Read the model definition and answer for the solid it produces. Units are mm, in the model's axes. Face numbers are marked on the shaded views. A direction names the side the tool comes from. Coordinates: 2 decimals unless noted, no trailing zeros. Write each loop counter-clockwise with the first axis right and the second up, starting at its lowest first coordinate (ties: lowest second). Pieces come first, ordered by that corner, then holes.
(1) The part is cut by section A-A, the plane x = 0. Determine the outline of the cut face in (y, z), and give its area (3 significant figures).
(2) The part is cut by section C-C, the plane z = 20. Determine the outline of the cut face in (x, y), and give its area (3 significant figures).
(3) The part is cut by section D-D, the plane x = -2.25. Determine the outline of the cut face in (y, z).
(4) The part is cut by section B-B, the plane y = 27.5. Determine the outline of the cut face in (x, z), and give its area (3 significant figures).
(5) Which of the six approach directions +Z, -Z, +X, -X, +Y, -Y give full straight-line access (tool end or side, diameter ignored) to the marked faces 1, 2 and 3?
(6) Given pin 1 (8 mm diameter, centred on y = 23, z = 13.5, fed in from +X), flat-ended and moving along its own axis, determine where the tip first touches the part or whether it passes through.
(7) Straight lines are drawn through the part: line 1 along Y through (x, z) = (-1, 21.5); line 2 along Y through (x, z) = (1, 9); line 3 along Z through (x, y) = (0, 17.5). For each, find the intervals that lie inside material, in ascending order.
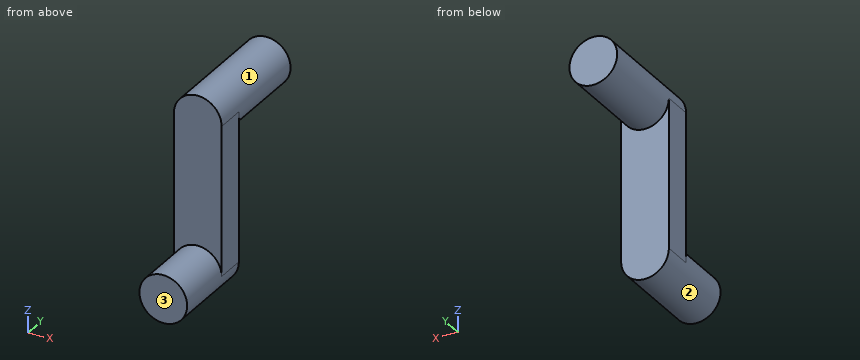
Autodesk Inventor part; units mm, degrees
ref_plane "YZ Plane" through (0, 0, 0) normal (1, 0, 0) x (0, 1, 0)
ref_plane "XZ Plane" through (0, 0, 0) normal (0, 1, 0) x (-1, 0, 0)
ref_plane "XY Plane" through (0, 0, 0) normal (0, 0, 1) x (1, 0, 0)
sketch "Sketch1" plane through (0, 0, 0) normal (0, 1, 0) x (-1, 0, 0)
  circle A0 centre (0, 0) radius 4
  dimension "d0" = 8
extrude "Extrusion1" add sketch "Sketch1" along normal blind 10
sketch "Sketch2" plane through (0, 10, 0) normal (0, 1, 0) x (1, 0, 0)
  circle A0 centre (0, 0) radius 4
  line L0 (4, 0) -> (-4, 0)
  line L1 (-4, 0) -> (-4, -25)
  line L2 (-4, -25) -> (4, -25)
  line L3 (4, -25) -> (4, 0)
  circle A1 centre (0, -25) radius 4
  dimension "d3" = 25
extrude "Extrusion2" add sketch "Sketch2" along normal blind 5
sketch "Sketch3" plane through (0, 15, 0) normal (0, 1, 0) x (1, 0, 0)
  arc A0 (-4, -25) -> (4, -25) centre (0, -25) ccw
  circle A1 centre (0, -25) radius 4
  point P0 (0, 0)
extrude "Extrusion3" add sketch "Sketch3" along normal blind 15
properties part number "Vevarm"
Computed:
1. outline: (0, -4) - (15, -4) - (15, 21) - (30, 21) - (30, 29) - (10, 29) - (10, 4) - (0, 4) - close
1. area: 365 mm2
2. outline: (-4, 10) - (4, 10) - (4, 15) - (-4, 15) - close
2. area: 40.0 mm2
3. outline: (0, -3.31) - (15, -3.31) - (15, 21.69) - (30, 21.69) - (30, 28.31) - (10, 28.31) - (10, 3.31) - (0, 3.31) - close
4. outline: circle Ø8 at (0, 25)
4. area: 50.3 mm2
5. face 1: +Y
5. face 2: -Y
5. face 3: +Z, -Z, +X, -X, -Y
6. pin 1: passes through
7. line 1: y = 10 to 30
7. line 2: y = 10 to 15
7. line 3: z = 21 to 29
